Design review of the part built by this model. Coordinates are the model's own, in mm. Coordinates: 2 decimals unless noted, no trailing zeros. Order: outer loops, then holes, each group sorted by start corner. A loop starts at its lowest first (then second) coordinate and runs counter-clockwise, first axis right, second up. Notation, with made-up numbers: M -14,-33.5 L 7,-33.5 A16 ccw 7,-17.5 Z; hole C -6.75,27 d3. An arc over 180 degrees is marked long. Answer in a Markdown table with one row per item.
Autodesk Inventor part; units mm, degrees
ref_plane "YZ Plane" through (0, 0, 0) normal (1, 0, 0) x (0, 1, 0)
ref_plane "XZ Plane" through (0, 0, 0) normal (0, 1, 0) x (-1, 0, 0)
ref_plane "XY Plane" through (0, 0, 0) normal (0, 0, 1) x (1, 0, 0)
sketch "Sketch1" plane through (0, 0, 0) normal (0, 0, 1) x (1, 0, 0)
  line L0 (-206.3501, 165.9986) -> (174.6499, 165.9986)
  line L1 (174.6499, 165.9986) -> (174.6499, -63.9984)
  line L2 (174.6499, -63.9984) -> (-206.3501, -63.9984)
  line L3 (-206.3501, -63.9984) -> (-206.3501, 165.9986)
  point P0 (0, 0)
  dimension "d0" = 381
  dimension "d1" = 229.997
extrude "Extrusion1" add sketch "Sketch1" along normal blind 6.35
hole "Hole1" at (-120.6251, 102.4986, 6.35) direction (0, 0, -1) diameter 76.2 end through all
pattern_linear "Rectangular Pattern1" count 3 spacing 101.6 along (1, 0, 0) count 2 spacing 101.6 along (0, -1, 0) of "Hole1"
hole "Hole2" at (-193.6501, -51.2984, 6.35) direction (0, 0, -1) diameter 3.175 end through all
pattern_linear "Rectangular Pattern2" count 14 spacing 25.4 along (1, 0, 0) of "Hole2"
hole "Hole3" at (161.9499, -51.2984, 6.35) direction (0, 0, -1) diameter 3.175 end through all
pattern_linear "Rectangular Pattern3" count 9 spacing 25.4 along (0, 1, 0) of "Hole2"
pattern_linear "Rectangular Pattern4" count 9 spacing 25.4 along (0, 1, 0) of "Hole3"
properties part number "Bottom"
(1) Add section A-A, the plane x = 53.5. Give the boundary of the cut face in (y, z), and give its area (3 significant figures).
Return value:
| item | result |
|---|---|
| outline | M -64,0 L -23.72,0 L -23.72,6.35 L -64,6.35 Z; M 25.52,0 L 77.88,0 L 77.88,6.35 L 25.52,6.35 Z; M 127.12,0 L 166,0 L 166,6.35 L 127.12,6.35 Z |
| area | 835 mm2 |
(2) Add section B-B, the plane y = 135.5. Give the boundary of the cut face in (x, z) (3 decimals), and give its area (3 significant figures).
Return value:
| item | result |
|---|---|
| outline | M -206.35,0 L -139.665,0 L -139.665,6.35 L -206.35,6.35 Z; M -101.585,0 L -38.065,0 L -38.065,6.35 L -101.585,6.35 Z; M 0.015,0 L 63.535,0 L 63.535,6.35 L 0.015,6.35 Z; M 101.615,0 L 174.65,0 L 174.65,6.35 L 101.615,6.35 Z |
| area | 1,690 mm2 |
(3) Insertion check: pin 1 Ø1.9 at (x, y) = (-168.25, -51.3) entering from -Z; pin 2 Ø3.5 at (x, y) = (-117.45, -51.3) entering from -Z. Each pin has a flat end and moves straight along its axis. Give the tip position at first contact, or say it passes through.
Return value:
| item | result |
|---|---|
| pin 1 | passes through |
| pin 2 | stops at z = 0 |
(4) Add section C-C, the plane z = 1.5. Give the number of separate pieces and of enclosed holes in the cut face, and give its area (3 significant figures).
Return value:
| item | result |
|---|---|
| separate pieces | 1 |
| enclosed holes | 37 |
| area | 60,000 mm2 |
(5) Add section D-D, the plane y = -12.5. Give the boundary of the cut face in (x, z).
Return value:
| item | result |
|---|---|
| outline | M -206.35,0 L -156.29,0 L -156.29,6.35 L -206.35,6.35 Z; M -84.96,0 L -54.69,0 L -54.69,6.35 L -84.96,6.35 Z; M 16.64,0 L 46.91,0 L 46.91,6.35 L 16.64,6.35 Z; M 118.24,0 L 174.65,0 L 174.65,6.35 L 118.24,6.35 Z |
(6) For line 1 along X through (y, z) = (101, 5); line 2 along Y through (x, z) = (82, 2.5); line 3 along X through (y, z) = (126, 6), list the stretches that pass through material, from the lowest coordinate up. Write a range as from..to.
Return value:
| item | result |
|---|---|
| line 1 | x = -206.35..-195.23, -192.07..-158.7, -82.55..-57.1, 19.05..44.5, 120.65..160.37, 163.53..174.65 |
| line 2 | y = -64..-37.2, 38.99..64.4, 140.59..166 |
| line 3 | x = -206.35..-195.16, -192.14..-150.61, -90.64..-49.01, 10.96..52.59, 112.56..160.44, 163.46..174.65 |
(7) Draft analysis for pull direction Y (two halves, no side actions). For faces 1 (the flat face through (-19, 53, 6.35)), 2 (the cylindrical face through (71.13, -35.44, 3.13)), state which applies: pulls with the +Y half, pulls with the -Y half, needs draft (parallel to the pull), parting line crosses it, or undercut.
Return value:
| item | result |
|---|---|
| face 1 | needs draft |
| face 2 | undercut |
